```python
from build123d import *

# Parameters (mm, degrees)
BOSS_EXTRUDE1_DEPTH       = 8
CUT_EXTRUDE2_DEPTH        = 21
BOSS_EXTRUDE2_DEPTH       = 3
BOSS_EXTRUDE5_DEPTH       = 5
SKETCH6_R                 = 1.6
CUT_EXTRUDE3_DEPTH        = 38.215588132
F_3_0MM_DOWEL_HOLE1_D     = 3
F_3_0MM_DOWEL_HOLE1_DEPTH = 5
F_3_0MM_DOWEL_HOLE1_TIP   = 0.901290929


with BuildPart() as part:
    # Sketch1 → Boss-Extrude1 (new body)
    with BuildSketch(Plane(origin=(0, 0, 0), x_dir=(0, 0, -1), z_dir=(1, 0, 0))):
        Polygon((0, 0), (0, 16), (-3, 16), (-3, 4), (-24, 4), (-24, 18), (-31, 18), (-31, 0), align=None)
    extrude(amount=-BOSS_EXTRUDE1_DEPTH)

    # Sketch5 → Cut-Extrude2 (cut)
    with BuildSketch(Plane.XY.offset(3)):
        Polygon((-8, 0), (-3, 0), (-5, 4), (-8, 4), align=None)
    extrude(amount=CUT_EXTRUDE2_DEPTH, mode=Mode.SUBTRACT)

    # Sketch8 → Boss-Extrude2 (add)
    with BuildSketch(Plane.XY.offset(3)):
        Polygon((-8, 4), (-5, 4), (-3, 0), (-8, 0), align=None)
    extrude(amount=BOSS_EXTRUDE2_DEPTH)

    # Sketch11 → Boss-Extrude5 (add)
    with BuildSketch(Plane.XZ):
        with BuildLine():
            Line((-10, 26), (-10, 33))
            Line((-10, 33), (-2, 33))
            ThreePointArc((-2, 33), (-0.585786438, 32.414213562), (0, 31))
            Line((0, 31), (-8, 31))
            Line((-8, 31), (-8, 24))
            ThreePointArc((-8, 24), (-9.414213562, 24.585786438), (-10, 26))
        make_face()
    extrude(amount=-BOSS_EXTRUDE5_DEPTH)

    # Sketch6 → Cut-Extrude3 (cut, through all)
    with BuildSketch(Plane.XY.offset(31)):
        with Locations((-4, 12)):
            Circle(SKETCH6_R)
    extrude(amount=-CUT_EXTRUDE3_DEPTH, mode=Mode.SUBTRACT)

    # Ø3.0mm Dowel Hole1
    with Locations(Plane(origin=(0, 0, 0), x_dir=(-1, 0, 0), z_dir=(0, -1, 0))):
        with Locations((5.715, -29)):
            Hole(F_3_0MM_DOWEL_HOLE1_D / 2, depth=F_3_0MM_DOWEL_HOLE1_DEPTH)
            with Locations((0, 0, -(F_3_0MM_DOWEL_HOLE1_DEPTH + F_3_0MM_DOWEL_HOLE1_TIP / 2))):  # 118° drill point
                Cone(0, F_3_0MM_DOWEL_HOLE1_D / 2, F_3_0MM_DOWEL_HOLE1_TIP, mode=Mode.SUBTRACT)


solid = part.part
```
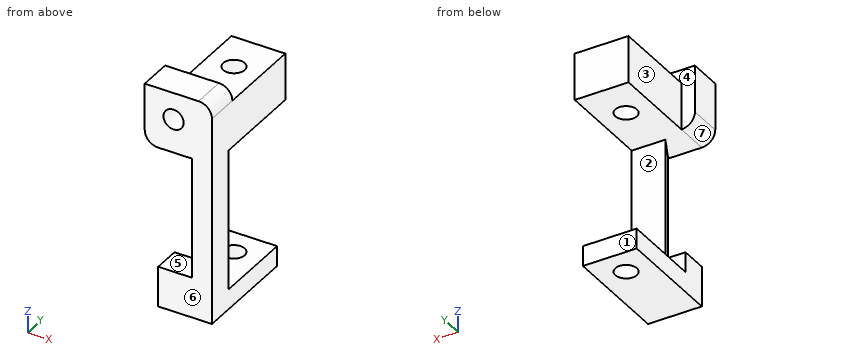
Input: part model. Units: mm. Frame: model coordinates. Face numbers are marked on the shaded views. A direction names the side the tool comes from. Coordinates: 2 decimals unless noted, no trailing zeros. Write each loop counter-clockwise with the first axis right and the second up, starting at its lowest first coordinate (ties: lowest second). Pieces come first, ordered by that corner, then holes. Notation, with made-up numbers: (89, 89) - (116, 89) arc R17 cw to (116, 110) - close; hole circle Ø9 at (85.25, 0). An arc over 180 degrees is marked (long way). Put each result on its own line as item: value. Start each with the question number.
1) Cut plane A-A (z = 27). Return the cut outline in (x, y), plus the area to 3 significant figures.
2) Mould query, pull axis Z, two halves, no side actions, for the marked faces 5, 6 and 7. Classes: pulls with the +Z half, pulls with the -Z half, needs draft (parallel to the pull), parting line crosses it, or undercut.
3) Contact query for flat-ended pins moving along their axis: pin 1 (1 mm diameter, centred on y = 6, z = 16.5, fed in from -X); pin 2 (1.8 mm diameter, centred on x = -5.715, z = 29, fed in from -Y); pin 3 (3 mm diameter, centred on x = -6, y = 15.5, fed in from +Z); pin 4 (1.5 mm diameter, centred on y = 3.5, z = 9.5, fed in from -X). Output: stop coordinate, or through.
4) Cut plane D-D (z = 17.5). Return the cut outline in (x, y).
5) Ray query, L1, parallel to X at y = 3.25, z = 29 (3 decimals); L2, parallel to Z at x = -3.75, y = 15.75; L3, parallel to Y at x = -4, z = 1.5. Return the intervals inside material, ascending.
6) Cut plane B-B (y = 9.5). Return the cut outline in (x, z), plus the area to 3 significant figures.
7) Reachability of the marked faces 1, 2, 3 and 4 from +Z, -Z, +X, -X, +Y, -Y: full face, straight path, thin tool, end or side. Return the list, or none.
8) Cut plane C-C (y = 12). Return the cut outline in (x, z).
Resolved:
1. outline: (-10, 0) - (0, 0) - (0, 18) - (-8, 18) - (-8, 5) - (-10, 5) - close; hole circle Ø3.2 at (-4, 12)
1. area: 146 mm2
2. face 5: undercut
2. face 6: needs draft
2. face 7: pulls with the -Z half
3. pin 1: passes through
3. pin 2: stops at y = 5.36
3. pin 3: stops at z = 31
3. pin 4: stops at x = -5
4. outline: (-5, 4) - (-3, 0) - (0, 0) - (0, 4) - close
5. L1: x = -10 to -7.215, -4.215 to 0
5. L2: z = 0 to 3, 24 to 31
5. L3: y = 0 to 10.4, 13.6 to 16
6. outline: (-8, 0) - (0, 0) - (0, 3) - (-8, 3) - close; (-8, 24) - (0, 24) - (0, 31) - (-8, 31) - close
6. area: 80.0 mm2
7. face 1: -Z, +X, -X, +Y
7. face 2: +X, -X, +Y
7. face 3: +Z, -Z, -X, +Y
7. face 4: +Z, -X, +Y
8. outline: (-8, 0) - (-5.6, 0) - (-5.6, 3) - (-8, 3) - close; (-8, 24) - (-5.6, 24) - (-5.6, 31) - (-8, 31) - close; (-2.4, 0) - (0, 0) - (0, 3) - (-2.4, 3) - close; (-2.4, 24) - (0, 24) - (0, 31) - (-2.4, 31) - close
